Part model, mm, in its own coordinate system. Face numbers are marked on the shaded views. Round coordinates to 2 decimals unless told otherwise and drop trailing zeros. Write each loop counter-clockwise with the first axis right and the second up, starting at its lowest first coordinate (ties: lowest second). Pieces come first, ordered by that corner, then holes. Notation, with made-up numbers: M 14,64.25 L 72,64.25 A3 ccw 72,68.25 Z; hole C 3,-2 d7. An arc over 180 degrees is marked long. Use a Markdown table: item, result. Add a question column.
1) Two-plate mould, pull along Y, no slides. Class the marked faces 1 and 2: released by +Y, released by -Y, zero draft, split by the parting line, or undercut.
2) Slice it at A-A on z = 5. Write the cut outline in (x, y), plus the area to 3 significant figures.
3) Wall check: probe 1 along Z at (x, y) = (-5, 2.25); probe 2 along X at (y, z) = (1.25, 4.5). Give the ranges that are in metal, low to high.
4) Slice it at B-B on x = -5.25. Write the cut outline in (y, z).
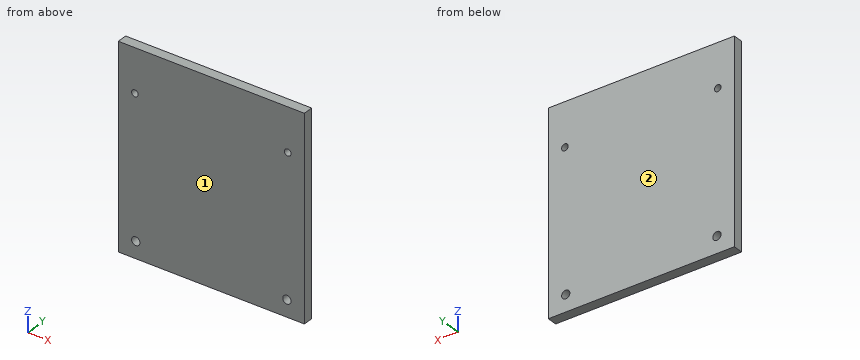
Autodesk Inventor part; units mm, degrees
ref_plane "YZ Plane" through (0, 0, 0) normal (1, 0, 0) x (0, 1, 0)
ref_plane "XZ Plane" through (0, 0, 0) normal (0, 1, 0) x (-1, 0, 0)
ref_plane "XY Plane" through (0, 0, 0) normal (0, 0, 1) x (1, 0, 0)
sketch "Sketch1" plane through (0, 0, 0) normal (0, 1, 0) x (-1, 0, 0)
  line L0 (0, 0) -> (56, 0)
  line L1 (56, 0) -> (56, 60)
  line L2 (56, 60) -> (0, 60)
  line L3 (0, 60) -> (0, 0)
  circle A0 centre (5.25, 5) radius 1.25
  circle A1 centre (5, 46.9993) radius 1
  line L4 (28, 60) -> (28, 0) construction
  circle A2 centre (50.75, 5) radius 1.25
  circle A3 centre (51, 46.9993) radius 1
  dimension "d0" = 56
  dimension "d1" = 60
  dimension "d4" = 2.5
  dimension "d5" = 5.25
  dimension "d6" = 5
  dimension "d7" = 2
  dimension "d8" = 5
  dimension "d9" = 42
extrude "Extrusion1" add sketch "Sketch1" along normal blind 3
properties part number "wall-front-outer-scaled"
Entries:
| question | item | result |
|---|---|---|
| 1 | face 1 | released by -Y |
| 1 | face 2 | released by +Y |
| 2 | outline | M -56,0 L -52,0 L -52,3 L -56,3 Z; M -49.5,0 L -6.5,0 L -6.5,3 L -49.5,3 Z; M -4,0 L 0,0 L 0,3 L -4,3 Z |
| 2 | area | 153 mm^2 |
| 3 | probe 1 | z = 0 to 3.78, 6.22 to 46, 48 to 60 |
| 3 | probe 2 | x = -56 to -51.9, -49.6 to -6.4, -4.1 to 0 |
| 4 | outline | M 0,0 L 3,0 L 3,3.75 L 0,3.75 Z; M 0,6.25 L 3,6.25 L 3,46.03 L 0,46.03 Z; M 0,47.97 L 3,47.97 L 3,60 L 0,60 Z |
